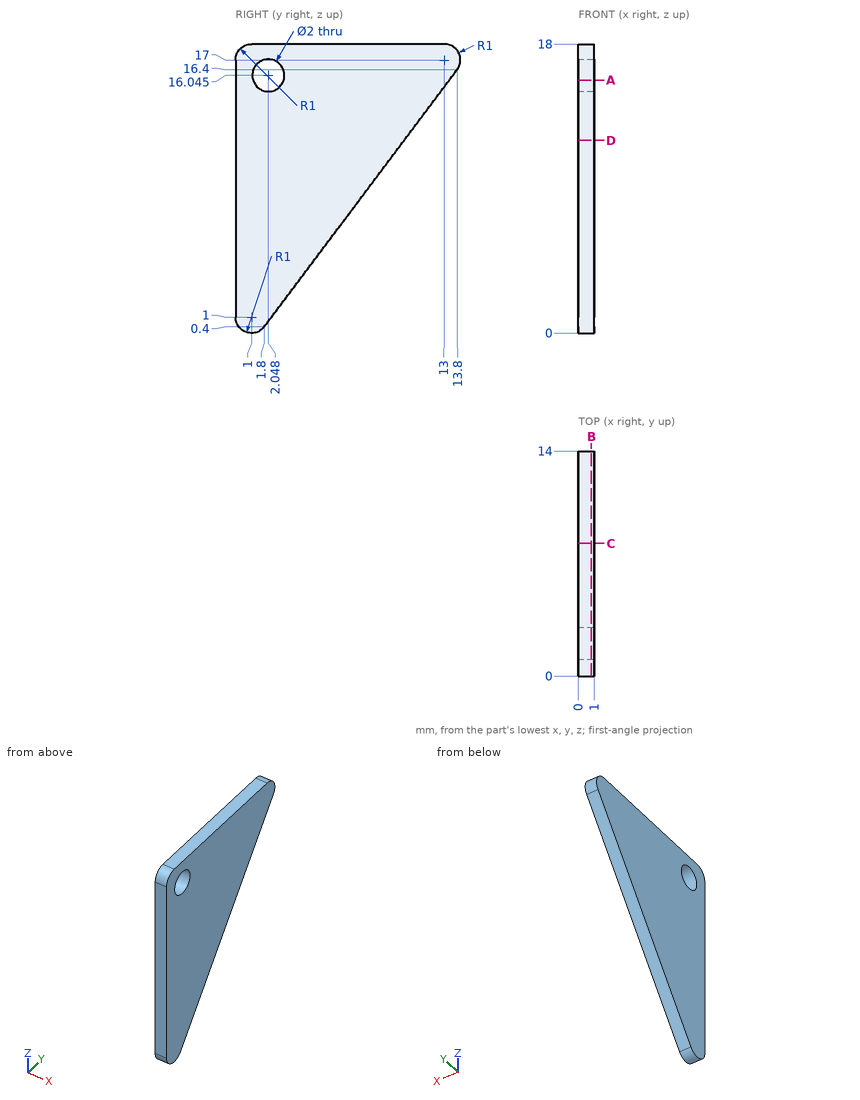
Source: three-view drawing plus pictorial views. Frame: mm from the lowest corner of the part. Give positions to 0.01 mm unless a question says otherwise; leave off trailing zeros. Write each loop counter-clockwise with the first axis right and the second up, starting at its lowest first coordinate (ties: lowest second). Pieces come first, ordered by that corner, then holes. Notation, with made-up numbers: (52, 27) - (108, 27) arc R24 ccw to (108, 53) - close; hole circle Ø5 at (-13, 55). An arc over 180 degrees is marked (long way). Write item = value, one per line. Start each with the question number.
1. Section query D-D, the plane z = 12. Output: boundary loops of the cut face in (x, y).
2. Section query C-C, the plane y = 8.25. Output: boundary loops of the cut face in (x, z).
3. First-contact query: pin 1 Ø2.5 at (y, z) = (2.05, 16.05) entering from +X. Flat tip, straight axial feed; report the tip coordinate or a pass-through.
4. Section query B-B, the plane x = 0.8. Output: boundary loops of the cut face in (y, z) (1 decimal).
5. Ray query, L1, parallel to Z at x = 0.6, y = 12; L2, parallel to Y at x = 0.45, z = 16.25 (1 decimal); L3, parallel to Y at x = 0.5, z = 16.5 (1 decimal). Return the intervals inside material, ascending.
6. Section query A-A, the plane z = 15.75. Output: boundary loops of the cut face in (x, y).
Check sheet entries:
q1.outline = (0, 0) - (1, 0) - (1, 10.5) - (0, 10.5) - close
q2.outline = (0, 9) - (1, 9) - (1, 18) - (0, 18) - close
q3.pin_1 = 1
q4.outline = (0, 1) arc R1 ccw to (1.8, 0.4) - (13.8, 16.4) arc R1 ccw to (13, 18) - (1, 18) arc R1 ccw to (0, 17) - close; hole circle Ø2 at (2, 16)
q5.L1 = 14 to 18
q5.L2 = 0 to 1.1, 3 to 13.7
q5.L3 = 0 to 1.2, 2.9 to 13.9
q6.outline = (0, 0) - (1, 0) - (1, 1.09) - (0, 1.09) - close; (0, 3) - (1, 3) - (1, 13.31) - (0, 13.31) - close
